from build123d import *

# Parameters (mm, degrees)
F0_W     = 35
F0_H     = 35
F0_W_2   = 20
F0_H_2   = 20
F1_DEPTH = 60
F2_R     = 5
F3_R     = 2
F4_DEPTH = 10


with BuildPart() as f1:
    # F0 (on Top) → F1 (new body)
    with BuildSketch(Plane.XY):
        Rectangle(F0_W, F0_H)
        Rectangle(F0_W_2, F0_H_2, mode=Mode.SUBTRACT)
    extrude(amount=F1_DEPTH)

    # F2
    f2_edges = [f1.edges().sort_by_distance(p)[0] for p in [
        (17.5, 17.5, 30),
        (-17.5, 17.5, 30),
        (17.5, -17.5, 30),
        (-17.5, -17.5, 30),
    ]]
    fillet(f2_edges, radius=F2_R)

    # F3 (on face) → F4 (cut)
    with BuildSketch(Plane.YZ.offset(17.5)):
        with Locations((0, 40)):
            Circle(F3_R)
        with Locations((0, 20)):
            Circle(F3_R)
    extrude(amount=-F4_DEPTH, mode=Mode.SUBTRACT)


solid = f1.part
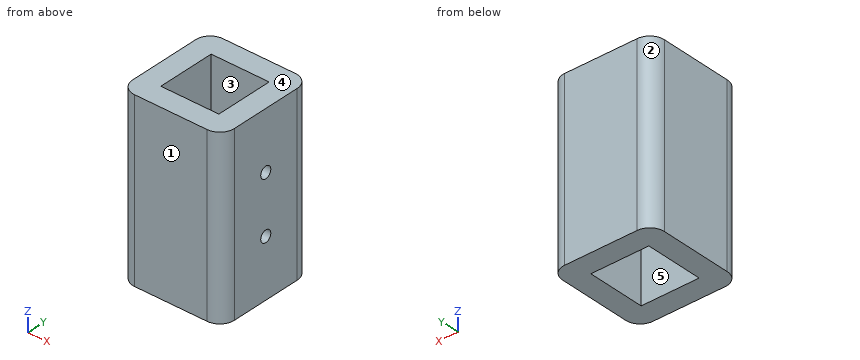
Model file for the job. Use its own axes, mm. Face numbers are marked on the shaded views. A direction names the side the tool comes from. Round coordinates to 2 decimals unless told otherwise and drop trailing zeros. Loops run counter-clockwise (first coordinate to the right, second up) from the corner with the lowest first, then second, coordinate; pieces in that order, holes last.
1. Band-saw the part on C-C, the plane z = 24.5. List the corners of the cut face in (x, y).
Check values:
outline: (-17.5, -12.5) arc R5 ccw to (-12.5, -17.5) - (12.5, -17.5) arc R5 ccw to (17.5, -12.5) - (17.5, 12.5) arc R5 ccw to (12.5, 17.5) - (-12.5, 17.5) arc R5 ccw to (-17.5, 12.5) - close; hole (-10, -10) - (10, -10) - (10, 10) - (-10, 10) - close
2. Mould opens along X. For the marked faces 1, 2 and 3 say: +X half, -X half, draft (parallel to the pull), parting line (faces both ways), or undercut.
Check values:
face 1: draft
face 2: -X half
face 3: undercut
3. Band-saw the part on B-B, the plane x = -9. List the corners of the cut face in (y, z), and give its area (3 significant figures).
Check values:
outline: (-17.5, 0) - (-10, 0) - (-10, 60) - (-17.5, 60) - close; (10, 0) - (17.5, 0) - (17.5, 60) - (10, 60) - close
area: 900 mm2
4. Band-saw the part on A-A, the plane y = 0. List the corners of the cut face in (x, z).
Check values:
outline: (-17.5, 0) - (-10, 0) - (-10, 60) - (-17.5, 60) - close; (10, 0) - (17.5, 0) - (17.5, 18) - (10, 18) - close; (10, 22) - (17.5, 22) - (17.5, 38) - (10, 38) - close; (10, 42) - (17.5, 42) - (17.5, 60) - (10, 60) - close
5. Tool access for the marked faces 4 and 5: list every direction of +Z, -Z, +X, -X, +Y, -Y with a clear straight run to the whole face (end or side of a thin tool).
Check values:
face 4: +Z, +X, -X, +Y, -Y
face 5: +Z, -Z
6. Wall check: probe 1 along Z at (x, y) = (15.25, 0); probe 2 along Y at (x, z) = (-6, 39). Give the ranges that are in metal, low to high.
Check values:
probe 1: z = 0 to 18, 22 to 38, 42 to 60
probe 2: y = -17.5 to -10, 10 to 17.5
